Part model, mm, in its own coordinate system. Face numbers are marked on the shaded views. A direction names the side the tool comes from. Give positions to 0.01 mm unless a question says otherwise; leave off trailing zeros. Order: outer loops, then holes, each group sorted by start corner. A loop starts at its lowest first (then second) coordinate and runs counter-clockwise, first axis right, second up.
1. Slice it at A-A on x = -9. List the corners of the cut face in (y, z), and give its area (3 significant figures).
2. Drop flat-ended pins along their axis: pin 1 Ø3.5 at (x, y) = (-6, 0) entering from +Z; pin 2 Ø1.2 at (y, z) = (-12.5, 2.5) entering from +X; pin 3 Ø6 at (y, z) = (8, 25) entering from +X; pin 4 Ø4 at (x, z) = (9.5, 7) entering from -Y. Give the stop position or say it passes through.
3. Mould opens along Z. For the marked faces 1, 2 and 3 say: +Z half, -Z half, draft (parallel to the pull), parting line (faces both ways), or undercut.
4. Probe line 1 (Y direction, x = -0.75, z = 7); line 2 (Z direction, x = -1.75, y = 2); line 3 (X direction, y = -14.5, z = 3.5). List the from-to ranges inside material, lowest first.
5. Slice it at B-B on z = 28.5. Give the number of separate pieces and of enclosed holes in the cut face, and give its area (3 significant figures).
6. Which spindle directions (+Z, -Z, +X, -X, +Y, -Y) get a long thin tool onto all of the face, cutting with end or side? Do the marked faces 4, 5 and 6. Say none if no direction does.
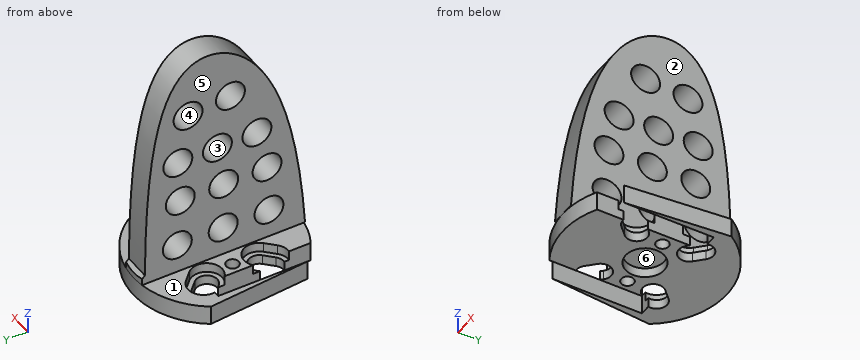
from build123d import *

# Parameters (mm, degrees)
SKETCH_2_R              = 1.3
EXTRUDE_1_DEPTH         = 4
CUT_EXTRUDE_1_DEPTH     = 2
EXTRUDE_START           = -2.75
EXTRUDE_2_DEPTH         = 5.5
CUT_EXTRUDE1_DEPTH      = 56.700937662
CUT_EXTRUDE1_DEPTH_BACK = 56.700937662
SKETCH_12_R             = 3
SKETCH1_R               = 4
CUT_EXTRUDE2_DEPTH      = 2


# Read off the part's stored shape, not the designer's step: 凸台-拉伸2
with BuildPart() as part:
    # 草图2 → 凸台-拉伸1 (new body)
    with BuildSketch(Plane.XY):
        with BuildLine():
            Line((-14.150895062, 9.420836955), (-12.3, -11.734990413))
            Line((-12.3, -11.734990413), (-12.3, 6.8))
            Line((-12.3, 6.8), (-10.126248664, 6.8))
            ThreePointArc((-10.126248664, 6.8), (-8.997025336, 9.159328805), (-6.410287771, 8.771557608))
            Line((-6.410287771, 8.771557608), (-4.642520818, 7.003790655))
            ThreePointArc((-4.642520818, 7.003790655), (-4.642520818, 3.892520818), (-7.753790655, 3.892520818))
            Line((-7.753790655, 3.892520818), (-8.2, 4.338730163))
            Line((-8.2, 4.338730163), (-8.2, -4.338730163))
            Line((-8.2, -4.338730163), (-7.753790655, -3.892520818))
            ThreePointArc((-7.753790655, -3.892520818), (-4.642520818, -3.892520818), (-4.642520818, -7.003790655))
            Line((-4.642520818, -7.003790655), (-6.410287771, -8.771557608))
            ThreePointArc((-6.410287771, -8.771557608), (-7.233498139, -9.29042366), (-8.2, -9.403434475))
            Line((-8.2, -9.403434475), (-8.2, -14.891608375))
            ThreePointArc((-8.2, -14.891608375), (0, -17), (8.2, -14.891608375))
            Line((8.2, -14.891608375), (8.2, -9.403434475))
            ThreePointArc((8.2, -9.403434475), (7.233498139, -9.29042366), (6.410287771, -8.771557608))
            Line((6.410287771, -8.771557608), (4.642520818, -7.003790655))
            ThreePointArc((4.642520818, -7.003790655), (4.642520818, -3.892520818), (7.753790655, -3.892520818))
            Line((7.753790655, -3.892520818), (8.2, -4.338730163))
            Line((8.2, -4.338730163), (8.2, 4.338730163))
            Line((8.2, 4.338730163), (7.753790655, 3.892520818))
            ThreePointArc((7.753790655, 3.892520818), (4.642520818, 3.892520818), (4.642520818, 7.003790655))
            Line((4.642520818, 7.003790655), (6.410287771, 8.771557608))
            ThreePointArc((6.410287771, 8.771557608), (8.997025336, 9.159328805), (10.126248664, 6.8))
            Line((10.126248664, 6.8), (12.3, 6.8))
            Line((12.3, 6.8), (12.3, -11.734990413))
            Line((12.3, -11.734990413), (14.150895062, 9.420836955))
            ThreePointArc((14.150895062, 9.420836955), (0, 17), (-14.150895062, 9.420836955))
        make_face()
        with Locations((-6, 0)):
            Circle(SKETCH_2_R, mode=Mode.SUBTRACT)
        with Locations((6, 0)):
            Circle(SKETCH_2_R, mode=Mode.SUBTRACT)
    extrude(amount=EXTRUDE_1_DEPTH)

    # 草图10 → 切除-拉伸1 (cut)
    with BuildSketch(Plane.XY.offset(4)):
        with BuildLine():
            Line((-5.703180989, 9.478664389), (-3.935414036, 7.710897436))
            ThreePointArc((-3.935414036, 7.710897436), (-3.935414036, 3.185414036), (-8.460897436, 3.185414036))
            Line((-8.460897436, 3.185414036), (-10.228664389, 4.953180989))
            ThreePointArc((-10.228664389, 4.953180989), (-10.228664389, 9.478664389), (-5.703180989, 9.478664389))
        make_face()
        with BuildLine():
            Line((-5.703180989, -9.478664389), (-3.935414036, -7.710897436))
            ThreePointArc((-3.935414036, -7.710897436), (-3.935414036, -3.185414036), (-8.460897436, -3.185414036))
            Line((-8.460897436, -3.185414036), (-10.228664389, -4.953180989))
            ThreePointArc((-10.228664389, -4.953180989), (-10.228664389, -9.478664389), (-5.703180989, -9.478664389))
        make_face()
        with BuildLine():
            Line((5.703180989, 9.478664389), (3.935414036, 7.710897436))
            ThreePointArc((3.935414036, 7.710897436), (3.935414036, 3.185414036), (8.460897436, 3.185414036))
            Line((8.460897436, 3.185414036), (10.228664389, 4.953180989))
            ThreePointArc((10.228664389, 4.953180989), (10.228664389, 9.478664389), (5.703180989, 9.478664389))
        make_face()
        with BuildLine():
            Line((5.703180989, -9.478664389), (3.935414036, -7.710897436))
            ThreePointArc((3.935414036, -7.710897436), (3.935414036, -3.185414036), (8.460897436, -3.185414036))
            Line((8.460897436, -3.185414036), (10.228664389, -4.953180989))
            ThreePointArc((10.228664389, -4.953180989), (10.228664389, -9.478664389), (5.703180989, -9.478664389))
        make_face()
    extrude(amount=-CUT_EXTRUDE_1_DEPTH, mode=Mode.SUBTRACT)

    # 凸台-拉伸2 outline → 凸台-拉伸2 (add)
    with BuildSketch(Plane(origin=(0, 0, 0), x_dir=(0, 0, -1), z_dir=(1, 0, 0)).offset(EXTRUDE_START)):
        with BuildLine():
            Line((-4, -17), (-4, 16.202251592))
            add(Edge.make_bspline(
                [(-4, 16.202251592), (-50.403204907, 16.202251592), (-54, 9.725618943), (-54, 4.360529693), (-54, -6.197938172), (-42.848798898, -14.485976771), (-4, -17)],
                knots=[0, 0, 0, 0, 0, 0, 0, 1, 1, 1, 1, 1, 1, 1], degree=6))
        make_face()
    extrude(amount=EXTRUDE_2_DEPTH)

    # 草图12 → Cut-Extrude1 (cut, two sides: drawn at the far end of the back side and taken through both)
    with BuildSketch(Plane(origin=(0, 0, 0), x_dir=(0, 0, -1), z_dir=(1, 0, 0)).offset(-CUT_EXTRUDE1_DEPTH_BACK)):
        with Locations((-10.089597621, 9.477228666)):
            Circle(SKETCH_12_R)
        with Locations((-10.089597621, -0.022771334)):
            Circle(SKETCH_12_R)
        with Locations((-10.089597621, -9.522771334)):
            Circle(SKETCH_12_R)
        with Locations((-20.089597621, 8.870444711)):
            Circle(SKETCH_12_R)
        with Locations((-20.089597621, -0.129555289)):
            Circle(SKETCH_12_R)
        with Locations((-20.089597621, -9.129555289)):
            Circle(SKETCH_12_R)
        with Locations((-29.034050933, 9.370090845)):
            Circle(SKETCH_12_R)
        with Locations((-29.034050933, 1.170090845)):
            Circle(SKETCH_12_R)
        with Locations((-29.034050933, -7.029909155)):
            Circle(SKETCH_12_R)
        with Locations((-39.034050933, 7.253595653)):
            Circle(SKETCH_12_R)
        with Locations((-39.868738586, -1.533288714)):
            Circle(SKETCH_12_R)
    extrude(amount=CUT_EXTRUDE1_DEPTH + CUT_EXTRUDE1_DEPTH_BACK, mode=Mode.SUBTRACT)

    # Chamfer1
    # the kernel refuses this chamfer: 2 mm, written as the material it adds along each edge
    with BuildSketch(Plane(origin=(-2.75, 16.202251592, 4), x_dir=(0, 0.9996220479086322, -0.02749111374520749), z_dir=(1, 0, 0))) as chamfer1_piece_1_section:
        with BuildLine():
            Line((2.052390471, 0), (-0.118013525, 2.043637132))
            Line((-0.118013525, 2.043637132), (-0.157992204, 2.042331311))
            ThreePointArc((-0.157992204, 2.042331311), (-0.069435245, 1.021504542), (-0.039984882, -0.001099645))
            Line((-0.039984882, -0.001099645), (0.001099645, -0.039984882))
            ThreePointArc((0.001099645, -0.039984882), (1.026519321, -0.011784294), (2.053490116, -0.039984882))
            Line((2.053490116, -0.039984882), (2.052390471, 0))
        make_face()
    chamfer1_piece_1 = extrude(amount=5.5, mode=Mode.PRIVATE)
    chamfer1_piece_1 = chamfer1_piece_1 & Plane(origin=(0, 0, 4.838799384), x_dir=(0.8324055918974517, 0.5541668797193253, 0), z_dir=(0, 0, -1)) * Cylinder(17, 20, mode=Mode.PRIVATE)
    add(chamfer1_piece_1)

    # Sketch1 → Cut-Extrude2 (cut)
    with BuildSketch(Plane(origin=(0, 0, 0), x_dir=(-1, 0, 0), z_dir=(0, 0, -1))):
        Circle(SKETCH1_R)
    extrude(amount=-CUT_EXTRUDE2_DEPTH, mode=Mode.SUBTRACT)


solid = part.part
Data:
1. outline: (9.16, 0) - (14.42, 0) - (14.42, 4) - (10.24, 4) - (10.24, 2) - (9.16, 2) - close
1. area: 18.9 mm2
2. pin 1: stops at z = 4
2. pin 2: stops at x = 8.2
2. pin 3: stops at x = 2.75
2. pin 4: passes through
3. face 1: +Z half
3. face 2: draft
3. face 3: undercut
4. line 1: y = -16.79 to 16.19
4. line 2: z = 2 to 7.87, 12.31 to 17.98, 22.2 to 26.15, 31.92 to 51
4. line 3: x = -8.2 to 8.2
5. separate pieces: 4
5. enclosed holes: 0
5. area: 60.7 mm2
6. face 4: +X, -X
6. face 5: +Z, -X, +Y, -Y
6. face 6: -Z
